```python
from build123d import *

# Parameters (mm, degrees)
EXTRUDE_2_DEPTH     = 1
EXTRUDE_3_DEPTH     = 37
SKETCH_3_W          = 2.5
SKETCH_3_H          = 25
EXTRUDE_4_DEPTH     = 30
SKETCH_4_W          = 10
SKETCH_4_H          = 15
EXTRUDE_5_DEPTH     = 26
CUT_EXTRUDE_1_REACH = 119.021
SKETCH_5_R          = 3.25


with BuildPart() as part:
    # Sketch 2 → Extrude 2 (new body)
    with BuildSketch(Plane(origin=(0, 0, 0), x_dir=(1, 0, 0), z_dir=(0, 1, 0))):
        Polygon((10, 15), (10, 10), (0, 10), (0, -10), (10, -10), (10, -15), (110, -15), (110, 15), align=None)
    extrude(amount=EXTRUDE_2_DEPTH)

    # Sketch 2_3 → Extrude 3 (add)
    with BuildSketch(Plane(origin=(0, 0, 0), x_dir=(1, 0, 0), z_dir=(0, 1, 0))):
        Polygon((10, 15), (10, 10), (0, 10), (0, -10), (10, -10), (10, -15), (110, -15), (110, 15), align=None)
        Polygon((12.5, 12.5), (107.5, 12.5), (107.5, -12.5), (12.5, -12.5), (12.5, -7.5), (2.5, -7.5), (2.5, 7.5), (12.5, 7.5), align=None, mode=Mode.SUBTRACT)
    extrude(amount=EXTRUDE_3_DEPTH)

    # Sketch 3 → Extrude 4 (add)
    with BuildSketch(Plane(origin=(0, 1, 0), x_dir=(1, 0, 0), z_dir=(0, 1, 0))):
        with Locations((24.25, 0)):
            Rectangle(SKETCH_3_W, SKETCH_3_H)
        with Locations((41.75, 0)):
            Rectangle(SKETCH_3_W, SKETCH_3_H)
        with Locations((59.25, 0)):
            Rectangle(SKETCH_3_W, SKETCH_3_H)
        with Locations((76.75, 0)):
            Rectangle(SKETCH_3_W, SKETCH_3_H)
        with Locations((94.25, 0)):
            Rectangle(SKETCH_3_W, SKETCH_3_H)
    extrude(amount=EXTRUDE_4_DEPTH)

    # Sketch 4 → Extrude 5 (add)
    with BuildSketch(Plane(origin=(0, 1, 0), x_dir=(1, 0, 0), z_dir=(0, 1, 0))):
        with Locations((7.5, 0)):
            Rectangle(SKETCH_4_W, SKETCH_4_H)
    extrude(amount=EXTRUDE_5_DEPTH)

    # Sketch 5 → Cut-Extrude 1 (cut, up to next)
    with BuildSketch(Plane.ZY, mode=Mode.PRIVATE) as cut_extrude_1_sk1:
        with Locations((0, 32)):
            Circle(SKETCH_5_R)
    cut_extrude_1_tool1 = extrude(cut_extrude_1_sk1.sketch, amount=-CUT_EXTRUDE_1_REACH, mode=Mode.PRIVATE) & part.part
    add(cut_extrude_1_tool1.solids().sort_by_distance((0, 32, 0))[0], mode=Mode.SUBTRACT)


solid = part.part
```
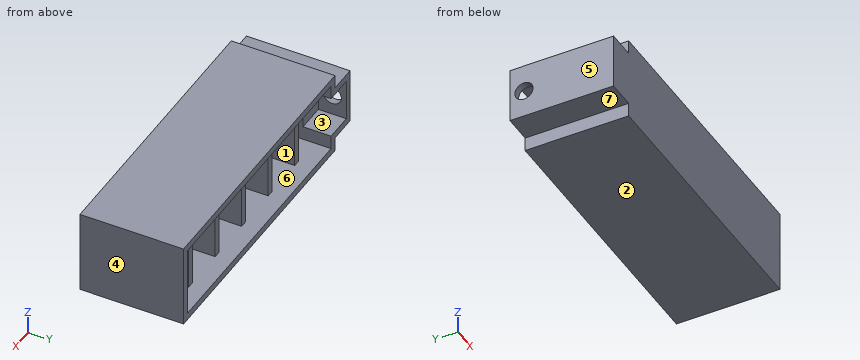
Part model, mm, in its own coordinate system. Face numbers are marked on the shaded views. A direction names the side the tool comes from. Round coordinates to 2 decimals unless told otherwise and drop trailing zeros. Loops run counter-clockwise (first coordinate to the right, second up) from the corner with the lowest first, then second, coordinate; pieces in that order, holes last.
1. Slice it at A-A (x = 89.5). Give the cut face in (y, z), and give its area (3 significant figures).
Solutions:
outline: (0, -15) - (37, -15) - (37, -12.5) - (1, -12.5) - (1, 12.5) - (37, 12.5) - (37, 15) - (0, 15) - close
area: 210 mm2
2. Two-plate mould, pull along X, no slides. Class the marked faces 1, 2, 3 and 4: pulls with the +X half, pulls with the -X half, needs draft (parallel to the pull), parting line crosses it, or undercut.
Solutions:
face 1: undercut
face 2: needs draft
face 3: undercut
face 4: pulls with the +X half
3. Flat gauge pins, fed straight in: pin 1 (12 mm diameter, centred on x = 82.5, z = 0.5, fed in from +Y); pin 2 (9.5 mm diameter, centred on x = 102.5, z = 5.5, fed in from +Y); pin 3 (4 mm diameter, centred on y = 22.5, z = -3, fed in from -X); pin 4 (3 mm diameter, centred on x = 7.5, y = 30, fed in from -Z). Where does each tip first touch, or does it go through?
Solutions:
pin 1: stops at y = 31
pin 2: stops at y = 1
pin 3: stops at x = 0
pin 4: stops at z = -10
4. Drill centre lines: line 1 along X through (y, z) = (35.5, 7); line 2 along Z through (x, y) = (62.5, 31.5); line 3 along Y through (x, z) = (0.65, 0). Where is each one in solid material? Low to high.
Solutions:
line 1: x = 0 to 2.5, 107.5 to 110
line 2: z = -15 to -12.5, 12.5 to 15
line 3: y = 0 to 28.75, 35.25 to 37
5. Slice it at C-C (y = 24.5). Count the separate pieces of the cut face and the enclosed holes in it, and give its area (3 significant figures).
Solutions:
separate pieces: 1
enclosed holes: 6
area: 1,140 mm2
6. 3-axis set-ups, long thin cutter, end or side, ignore diameter. For the marked faces 5, 6 and 7: which of +Z, -Z, +X, -X, +Y, -Y reach the whole face in a straight line?
Solutions:
face 5: +Z, -Z, -X, +Y, -Y
face 6: +Y
face 7: -Z, -X, +Y, -Y
